Check sheet for the modelled part. Datum: model origin and axes. Units: mm. Give positions to 0.01 mm unless a question says otherwise; leave off trailing zeros. Write each loop counter-clockwise with the first axis right and the second up, starting at its lowest first coordinate (ties: lowest second). Pieces come first, ordered by that corner, then holes. Notation, with made-up numbers: (-9, 44) -> (32, 44) arc R21 ccw to (32, 69) -> close; hole circle Ø6 at (83.5, 52). An arc over 180 degrees is marked (long way). Use a Markdown table: item, result. Add a question column.
1. Scan lines: probe 1 along X at (y, z) = (0.9, 14); probe 2 along Z at (x, y) = (-18, 2.45); probe 3 along X at (y, z) = (0.85, 6.35). Record each from-to range of solid material in increasing order. Write a range as [from, to].
2. Cross-section at B-B (z = 6.35). Enter the section's corners in (x, y), then the cut area to 3 significant figures.
3. Gauge pin test, flat ends, axial feed: P1, Ø5.5, axis at x = 15.875, z = 6.35, coming from the +Y side; P2, Ø1.5, axis at x = 15, z = -4.5, coming from the -Y side. Record the tip position at first contact, or that the pin passes through.
4. Cross-section at D-D (z = -29). Enter the section's corners in (x, y).
5. Cross-section at C-C (y = 0.9). Count the separate pieces of the cut face and the enclosed holes in it, then the cut area to 3 significant figures.
6. Cross-section at A-A (z = -11). Enter the section's corners in (x, y).
from build123d import *

# Parameters (mm, degrees)
BOSS_EXTRUDE1_OUTLINE_W   = 57.5056
BOSS_EXTRUDE1_OUTLINE_H   = 101.6
BOSS_EXTRUDE1_OUTLINE_W_2 = 5.842
BOSS_EXTRUDE1_OUTLINE_H_2 = 12.6
BOSS_EXTRUDE1_DEPTH       = 3.0988
SKETCH2_R                 = 1.7526
CUT_EXTRUDE1_DEPTH        = 59.454820753
FILLET1_R                 = 6.35
SKETCH3_W                 = 58.835231844
SKETCH3_H                 = 12.7
CUT_EXTRUDE2_DEPTH        = 59.454820753
FILLET2_R                 = 2.54
SKETCH4_W                 = 76.889579371
SKETCH4_H                 = 12.7
CUT_EXTRUDE3_DEPTH        = 59.454820895
FILLET3_R                 = 6.35


# Read off the part's stored shape, not the designer's step: Boss-Extrude1
with BuildPart() as part:
    # Boss-Extrude1 outline → Boss-Extrude1 (new body)
    with BuildSketch(Plane(origin=(0, 0, 0), x_dir=(1, 0, 0), z_dir=(0, 1, 0))):
        Rectangle(BOSS_EXTRUDE1_OUTLINE_W, BOSS_EXTRUDE1_OUTLINE_H)
        with Locations((-15.875, -19.1)):
            Rectangle(BOSS_EXTRUDE1_OUTLINE_W_2, BOSS_EXTRUDE1_OUTLINE_H_2, mode=Mode.SUBTRACT)
        with Locations((15.875, -19.1)):
            Rectangle(BOSS_EXTRUDE1_OUTLINE_W_2, BOSS_EXTRUDE1_OUTLINE_H_2, mode=Mode.SUBTRACT)
        with Locations((-15.875, 6.4)):
            Rectangle(BOSS_EXTRUDE1_OUTLINE_W_2, BOSS_EXTRUDE1_OUTLINE_H_2, mode=Mode.SUBTRACT)
        with Locations((15.875, 6.4)):
            Rectangle(BOSS_EXTRUDE1_OUTLINE_W_2, BOSS_EXTRUDE1_OUTLINE_H_2, mode=Mode.SUBTRACT)
    extrude(amount=BOSS_EXTRUDE1_DEPTH)

    # Sketch2 → Cut-Extrude1 (cut, through all)
    with BuildSketch(Plane(origin=(0, 3.0988, 0), x_dir=(1, 0, 0), z_dir=(0, 1, 0))):
        with Locations(Location((-15.875, -6.35, 0), (0, 0, 270))):
            Circle(SKETCH2_R)
        with Locations(Location((15.875, -6.35, 0), (0, 0, 270))):
            Circle(SKETCH2_R)
        Polygon((18.796, 50.8), (28.7528, 25.4), (28.7528, 50.8), align=None)
        Polygon((28.7528, -38.1), (18.796, -50.8), (28.7528, -50.8), align=None)
        Polygon((-28.7528, -50.8), (-18.796, -50.8), (-28.7528, -38.1), align=None)
        Polygon((-28.7528, 50.8), (-28.7528, 25.4), (-18.796, 50.8), align=None)
    extrude(amount=-CUT_EXTRUDE1_DEPTH, mode=Mode.SUBTRACT)

    # Fillet1
    fillet1_edges = [part.edges().sort_by_distance(p)[0] for p in [
        (-28.7528, 1.5494, 38.1),
        (-28.7528, 1.5494, -25.4),
        (-18.796, 1.5494, -50.8),
        (28.7528, 1.5494, -25.4),
        (18.796, 1.5494, -50.8),
        (18.796, 1.5494, 50.8),
        (28.7528, 1.5494, 38.1),
        (-18.796, 1.5494, 50.8),
    ]]
    fillet(fillet1_edges, radius=FILLET1_R)

    # Sketch3 → Cut-Extrude2 (cut, through all)
    with BuildSketch(Plane(origin=(0, 0, 0), x_dir=(-1, 0, 0), z_dir=(0, -1, 0))):
        with Locations((0.664815922, -44.45)):
            Rectangle(SKETCH3_W, SKETCH3_H)
    extrude(amount=-CUT_EXTRUDE2_DEPTH, mode=Mode.SUBTRACT)

    # Fillet2
    fillet2_edges = [part.edges().sort_by_distance(p)[0] for p in [
        (-28.362298152, 1.5494, 38.1),
        (28.362298152, 1.5494, 38.1),
    ]]
    fillet(fillet2_edges, radius=FILLET2_R)

    # Sketch4 → Cut-Extrude3 (cut, through all)
    with BuildSketch(Plane(origin=(0, 0, 0), x_dir=(-1, 0, 0), z_dir=(0, -1, 0))):
        with Locations((3.167610928, 44.45)):
            Rectangle(SKETCH4_W, SKETCH4_H)
    extrude(amount=-CUT_EXTRUDE3_DEPTH, mode=Mode.SUBTRACT)

    # Fillet3
    fillet3_edges = [part.edges().sort_by_distance(p)[0] for p in [
        (-23.7744, 1.5494, -38.1),
        (23.7744, 1.5494, -38.1),
    ]]
    fillet(fillet3_edges, radius=FILLET3_R)


solid = part.part
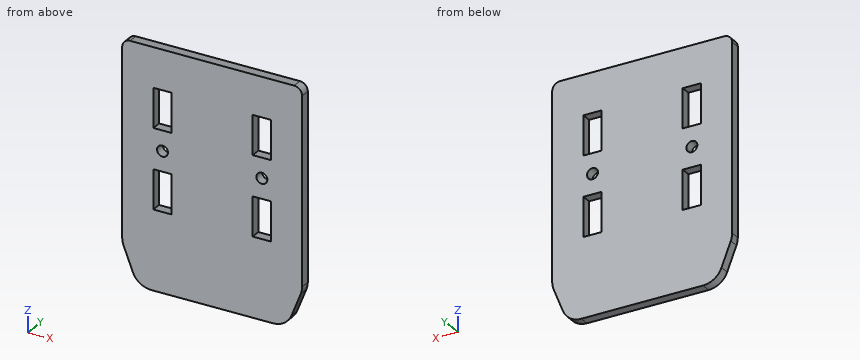
Worked answers:
| question | item | result |
|---|---|---|
| 1 | probe 1 | x = [-28.75, -18.8], [-12.95, 12.95], [18.8, 28.75] |
| 1 | probe 2 | z = [-38.1, -12.7], [-0.1, 12.8], [25.4, 38.1] |
| 1 | probe 3 | x = [-28.75, -17.63], [-14.12, 14.12], [17.63, 28.75] |
| 2 | outline | (-28.75, 0) -> (-17.63, 0) -> (-17.63, 3.1) -> (-28.75, 3.1) -> close; (-14.12, 0) -> (14.12, 0) -> (14.12, 3.1) -> (-14.12, 3.1) -> close; (17.63, 0) -> (28.75, 0) -> (28.75, 3.1) -> (17.63, 3.1) -> close |
| 2 | area | 156 mm² |
| 3 | P1 | stops at y = 3.1 |
| 3 | P2 | passes through |
| 4 | outline | (-27.34, 0) -> (27.34, 0) -> (27.34, 3.1) -> (-27.34, 3.1) -> close |
| 5 | separate pieces | 1 |
| 5 | enclosed holes | 6 |
| 5 | area | 4,000 mm² |
| 6 | outline | (-28.75, 0) -> (-18.8, 0) -> (-18.8, 3.1) -> (-28.75, 3.1) -> close; (-12.95, 0) -> (12.95, 0) -> (12.95, 3.1) -> (-12.95, 3.1) -> close; (18.8, 0) -> (28.75, 0) -> (28.75, 3.1) -> (18.8, 3.1) -> close |
